Could you check a few things on this drawing? It's one solid part, dimensions in mm from its lowest x, y, z. Give positions to 0.01 mm unless a question says otherwise; leave off trailing zeros. Loops run counter-clockwise (first coordinate to the right, second up) from the corner with the lowest first, then second, coordinate; pieces in that order, holes last. Notation, with made-up numbers: (-27, 50.5) - (-19, 50.5) arc R35 ccw to (-19, 82.5) - close; hole circle Ø7 at (-9, 23.5). An arc over 180 degrees is marked (long way). Write item = value, one per line.
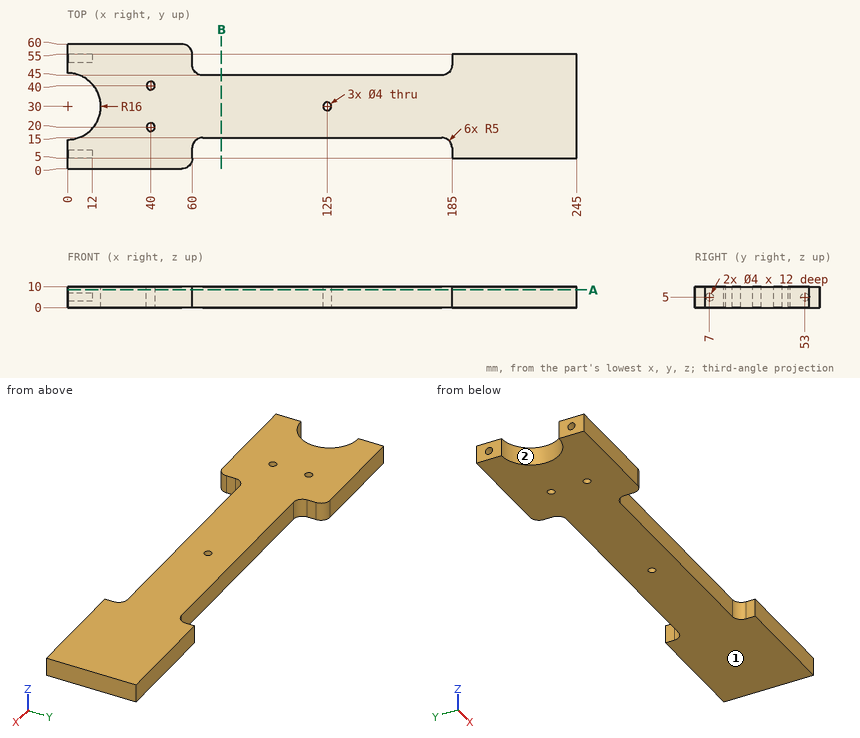
Q1. I need wall thicknesses on L1, parallel to Y at x = 40, z = 7.25; L2, parallel to X at y = 7, z = 9; L3, parallel to Y at x = 125, z = 5.25. Which ranges of each line are inside material? Lowest first, please.
Output:
L1 = 0 to 18, 22 to 38, 42 to 60
L2 = 0 to 60, 185 to 245
L3 = 15 to 28, 32 to 45
Q2. Imagine slicing it at A-A, the plane z = 8.5. Write out the boundary of the cut face in (x, y), then the cut area to 3 significant figures.
Output:
outline = (0, 0) - (55, 0) arc R5 ccw to (60, 5) - (60, 10) arc R5 cw to (65, 15) - (180, 15) arc R5 cw to (185, 10) - (185, 5) - (245, 5) - (245, 55) - (185, 55) - (185, 50) arc R5 cw to (180, 45) - (65, 45) arc R5 cw to (60, 50) - (60, 55) arc R5 ccw to (55, 60) - (0, 60) - (0, 46) arc R16 cw to (0, 14) - close; hole circle Ø4 at (40, 20); hole circle Ø4 at (40, 40); hole circle Ø4 at (125, 30)
area = 9,920 mm2
Q3. For pin 1 (2 mm diameter, centred on y = 7, z = 4.5, fed in from -X); pin 2 (3 mm diameter, centred on x = 96.5, z = 7, fed in from -Y), each with a flat end and sliding along its axis, tell me the tip position at first contact or that it passes through.
Output:
pin_1 = 12
pin_2 = 15
Q4. We'd pull the mould along Y, two halves only. Please class the marked faces 1 and 2: released by +Y, released by -Y, zero draft, split by the parting line, or undercut.
Output:
face_1 = zero draft
face_2 = undercut
Q5. Imagine slicing it at B-B, the plane x = 74. Write out the boundary of the cut face in (y, z).
Output:
outline = (15, 0) - (45, 0) - (45, 10) - (15, 10) - close
